Design review of the part built by this model. Coordinates are the model's own, in mm. Coordinates: 2 decimals unless noted, no trailing zeros. Loops run counter-clockwise (first coordinate to the right, second up) from the corner with the lowest first, then second, coordinate; pieces in that order, holes last. Notation, with made-up numbers: M -33,51.5 L 24,51.5 A26 cw 24,65.5 Z; hole C 78,6 d9. An arc over 180 degrees is marked long. Put each result on its own line as item: value. Start each with the question number.
(1) For probe 1 along Y at (x, z) = (27.75, -2.25); probe 2 along Y at (x, z) = (-27.75, -2.15); probe 3 along X at (y, z) = (29.75, -2), list the stretches that pass through material, from the lowest coordinate up. Write a range as [from, to].
(2) Clearance check with flat-ended pins moving along their axes: pin 1 (2.5 mm diameter, centred on x = 27.75, y = -29.75, fed in from +Z); pin 2 (1.6 mm diameter, centred on x = 29, y = 28.5, fed in from -Z). State where each tip first meets the part, or that it passes through.
(3) Take a section at A-A, the plane x = 20. Give the boundary of the cut face in (y, z), then the cut area to 4 significant figures.
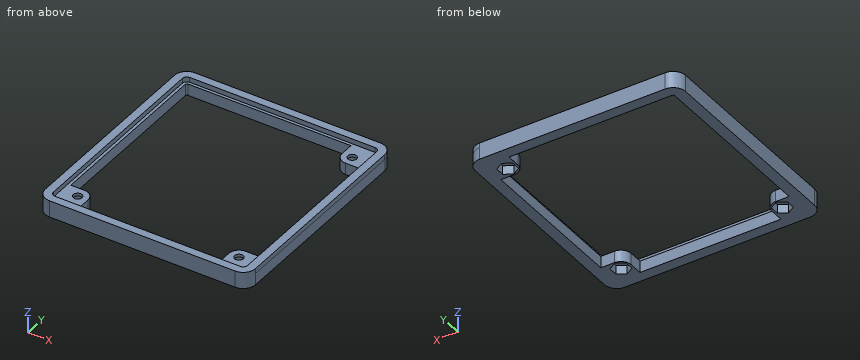
```python
from build123d import *

# Parameters (mm, degrees)
PAD007_DEPTH      = 1.5
PAD007_DEPTH_BACK = 0.2
SKETCH008_R       = 1.5
PAD008_DEPTH      = 4
POCKET006_DEPTH   = 3


with BuildPart() as part:
    # Sketch007 → Pad007 (new body, two sides)
    with BuildSketch(Plane.XY) as pad007_sk:
        with BuildLine():
            ThreePointArc((-31.9, 38.15), (-34.905204, 36.905204), (-36.15, 33.9))
            Line((-36.15, -33.9), (-36.15, 33.9))
            ThreePointArc((-36.15, -33.9), (-34.905204, -36.905204), (-31.9, -38.15))
            Line((31.9, -38.15), (-31.9, -38.15))
            ThreePointArc((31.9, -38.15), (34.905204, -36.905204), (36.15, -33.9))
            Line((36.15, 33.9), (36.15, -33.9))
            ThreePointArc((36.15, 33.9), (34.905204, 36.905204), (31.9, 38.15))
            Line((-31.9, 38.15), (31.9, 38.15))
        make_face()
        with BuildLine():
            ThreePointArc((-31.9, 35.4), (-32.96066, 34.96066), (-33.4, 33.9))
            Line((-33.4, -33.9), (-33.4, 33.9))
            ThreePointArc((-33.4, -33.9), (-32.96066, -34.96066), (-31.9, -35.4))
            Line((31.9, -35.4), (-31.9, -35.4))
            ThreePointArc((31.9, -35.4), (32.96066, -34.96066), (33.4, -33.9))
            Line((33.4, 33.9), (33.4, -33.9))
            ThreePointArc((33.4, 33.9), (32.96066, 34.96066), (31.9, 35.4))
            Line((-31.9, 35.4), (31.9, 35.4))
        make_face(mode=Mode.SUBTRACT)
    extrude(amount=-PAD007_DEPTH)
    extrude(pad007_sk.sketch, amount=PAD007_DEPTH_BACK)

    # Sketch008 → Pad008 (join)
    with BuildSketch(Plane(origin=(0, 0, -1.5), x_dir=(-1, 0, 0), z_dir=(0, 0, -1))):
        with BuildLine():
            ThreePointArc((-31.9, 38.15), (-34.869436, 36.94055), (-36.14881, 34.000563))
            Line((-36.15, -33.9), (-36.14881, 34.000563))
            ThreePointArc((-36.15, -33.9), (-34.905204, -36.905204), (-31.9, -38.15))
            Line((31.9, -38.15), (-31.9, -38.15))
            ThreePointArc((31.9, -38.15), (34.905204, -36.905204), (36.15, -33.9))
            Line((36.15, 33.9), (36.15, -33.9))
            ThreePointArc((36.15, 33.9), (34.905204, 36.905204), (31.9, 38.15))
            Line((-31.9, 38.15), (31.9, 38.15))
        make_face()
        with Locations((-27.75, 29.75)):
            Circle(SKETCH008_R, mode=Mode.SUBTRACT)
        with Locations((-27.75, -29.75)):
            Circle(SKETCH008_R, mode=Mode.SUBTRACT)
        with Locations((27.75, -29.75)):
            Circle(SKETCH008_R, mode=Mode.SUBTRACT)
        with BuildLine():
            ThreePointArc((-27.75, 26.25), (-25.275126, 27.275126), (-24.25, 29.75))
            Line((-24.25, 29.75), (-24.25, 34.4))
            Line((-24.25, 34.4), (31.9, 34.4))
            ThreePointArc((32.4, 33.9), (32.253553, 34.253553), (31.9, 34.4))
            Line((32.4, 33.9), (32.4, -26.25))
            Line((27.75, -26.25), (32.4, -26.25))
            ThreePointArc((27.75, -26.25), (25.275126, -27.275126), (24.25, -29.75))
            Line((24.25, -29.75), (24.25, -34.4))
            Line((-24.25, -34.4), (24.25, -34.4))
            Line((-24.25, -34.4), (-24.25, -29.75))
            ThreePointArc((-24.25, -29.75), (-25.275126, -27.275126), (-27.75, -26.25))
            Line((-32.4, -26.25), (-27.75, -26.25))
            Line((-32.4, 26.25), (-32.4, -26.25))
            Line((-32.4, 26.25), (-27.75, 26.25))
        make_face(mode=Mode.SUBTRACT)
    extrude(amount=PAD008_DEPTH)

    # Sketch021 → Pocket006 (cut)
    with BuildSketch(Plane(origin=(0, 0, -5.5), x_dir=(-1, 0, 0), z_dir=(0, 0, -1))):
        Polygon((-25, 28.162287), (-25, 31.337713), (-27.75, 32.925426), (-30.5, 31.337713), (-30.5, 28.162287), (-27.75, 26.574574), align=None)
        Polygon((-25, -31.337713), (-25, -28.162287), (-27.75, -26.574574), (-30.5, -28.162287), (-30.5, -31.337713), (-27.75, -32.925426), align=None)
        Polygon((30.5, -31.337713), (30.5, -28.162287), (27.75, -26.574574), (25, -28.162287), (25, -31.337713), (27.75, -32.925426), align=None)
    extrude(amount=-POCKET006_DEPTH, mode=Mode.SUBTRACT)


solid = part.part
```
Computed values:
1. probe 1: y = [-38.15, -31.25], [-28.25, -26.25], [26.25, 28.25], [31.25, 38.15]
1. probe 2: y = [-38.15, -31.25], [-28.25, -26.25], [34.4, 38.15]
1. probe 3: x = [-36.15, -32.4], [24.25, 26.25], [29.25, 36.15]
2. pin 1: passes through
2. pin 2: stops at z = -2.5
3. outline: M -38.15,-5.5 L -34.4,-5.5 L -34.4,-1.5 L -35.4,-1.5 L -35.4,0.2 L -38.15,0.2 Z; M 34.4,-5.5 L 38.15,-5.5 L 38.15,0.2 L 35.4,0.2 L 35.4,-1.5 L 34.4,-1.5 Z
3. area: 39.35 mm^2
